Work out the finished part from the listing and answer in its coordinate system (mm). Face numbers are marked on the shaded views. A direction names the side the tool comes from. Give positions to 0.01 mm unless a question says otherwise; leave off trailing zeros. Loops run counter-clockwise (first coordinate to the right, second up) from the corner with the lowest first, then second, coordinate; pieces in that order, holes last. Notation, with made-up numbers: (18, 79.5) - (72, 79.5) arc R21 cw to (72, 116.5) - close; hole circle Ø3 at (-6, 4.5). An arc over 180 degrees is marked (long way). One line per item, written item: value.
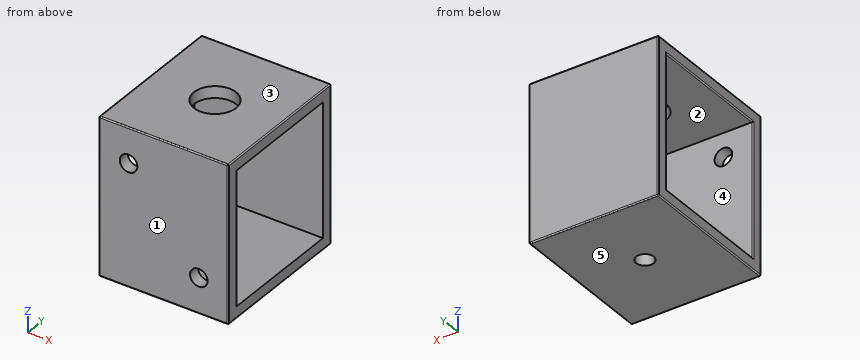
Autodesk Inventor part; units mm, degrees
ref_plane "YZ Plane" through (0, 0, 0) normal (1, 0, 0) x (0, 1, 0)
ref_plane "XZ Plane" through (0, 0, 0) normal (0, 1, 0) x (-1, 0, 0)
ref_plane "XY Plane" through (0, 0, 0) normal (0, 0, 1) x (1, 0, 0)
sketch "Sketch1" plane through (0, 0, 0) normal (0, 1, 0) x (-1, 0, 0)
  line L0 (11.5005, 11.58) -> (-10.5995, 11.58)
  line L1 (-10.5995, 11.58) -> (-10.5995, -15.22)
  line L2 (-10.5995, -15.22) -> (11.5005, -15.22)
  line L3 (11.5005, -15.22) -> (11.5005, 11.58)
  point P0 (0, 0)
  dimension "d0" = 22.1
  dimension "d1" = 26.8
extrude "Extrusion1" add sketch "Sketch1" along normal blind 25.4
shell "Shell1" thickness 2 removed faces 2 at (-11.5005, 8.4667, -6.2867) at (10.5995, 8.4667, 2.6466)
sketch "Sketch2" plane through (0, 0, 0) normal (0, -1, 0) x (1, 0, 0)
  line L0 (-11.5005, 11.58) -> (10.5995, 11.58)
  line L1 (-0.4505, 11.58) -> (-0.4505, -15.22)
  line L2 (10.5995, -15.22) -> (-11.5005, -15.22)
  circle A0 centre (-0.4505, -1.82) radius 9.5
  circle A1 centre (-6.4505, 5.5454) radius 1.5
  circle A2 centre (5.5495, -9.1855) radius 1.5
  point P0 (0, 0)
  dimension "d4" = 19
  dimension "d5" = 3
  dimension "d6" = 3
  dimension "d7" = 6
  dimension "d8" = 12
extrude "Extrusion2" cut sketch "Sketch2" against normal up to next contours A1 A0 | A0 A1 | A2 A0 | A0 A2
sketch "Sketch3" plane through (-11.5005, 0, 11.58) normal (0, 0, 1) x (1, 0, 0)
  line L0 (22.1, 0) -> (0, 0)
  line L1 (11.05, 0) -> (11.05, 25.4)
  line L2 (0, 25.4) -> (22.1, 25.4)
  circle A0 centre (11.05, 12.7) radius 3.6
  point P0 (11.5005, 0)
  dimension "d12" = 7.2
extrude "Extrusion3" cut sketch "Sketch3" against normal up to next
sketch "Sketch4" plane through (10.5995, 0, -15.22) normal (0, 0, -1) x (-1, 0, 0)
  line L0 (0, 25.4) -> (22.1, 25.4)
  line L1 (11.05, 25.4) -> (11.05, 0)
  line L2 (22.1, 0) -> (0, 0)
  circle A0 centre (11.05, 12.7) radius 1.5
  point P0 (10.5995, 0)
  dimension "d15" = 3
extrude "Extrusion4" cut sketch "Sketch4" against normal up to next
fillet "Fillet1" radius 0.2 16 edges at (-11.5005, 12.7, 11.58) (-0.4505, 0, 11.58) (10.5995, 12.7, 11.58) (10.5995, 0, -1.82) (-11.5005, 0, -1.82) (-0.4505, 0, -15.22) (10.5995, 12.7, -15.22) (-11.5005, 12.7, -15.22) (-0.4505, 25.4, -15.22) (-11.5005, 25.4, -1.82) (-0.4505, 25.4, 11.58) (10.5995, 25.4, -1.82) (-11.5005, 12.7, -13.22) (-11.5005, 2, -1.82) (-11.5005, 12.7, 9.58) (-11.5005, 23.4, -1.82)
properties part number "Solenoid_shell"
1. Section A-A (y = 12.7) is taken. Write down the section's boundary in (x, z).
Output:
outline: (-11.5, -15.02) arc R0.2 ccw to (-11.3, -15.22) - (-1.95, -15.22) - (-1.95, -13.22) - (-11.3, -13.22) arc R0.2 ccw to (-11.5, -13.42) - close; (-11.5, 9.78) arc R0.2 ccw to (-11.3, 9.58) - (-4.05, 9.58) - (-4.05, 11.58) - (-11.3, 11.58) arc R0.2 ccw to (-11.5, 11.38) - close; (1.05, -15.22) - (10.4, -15.22) arc R0.2 ccw to (10.6, -15.02) - (10.6, -13.22) - (1.05, -13.22) - close; (3.15, 9.58) - (10.6, 9.58) - (10.6, 11.38) arc R0.2 ccw to (10.4, 11.58) - (3.15, 11.58) - close
2. The mould has two halves that part along Z. Classify the marked faces 1, 2 and 3: released by +Z, released by -Z, zero draft, split by the parting line, or undercut.
Output:
face 1: zero draft
face 2: undercut
face 3: released by +Z
3. For the marked faces 4 and 5, determine the directions among +Z, -Z, +X, -X, +Y, -Y from which every point of the face is accessible in a straight line to the end or side of a thin tool.
Output:
face 4: +X, -X
face 5: -Z, +X, -X, +Y, -Y
4. Section C-C (x = 3.5) is taken. Write down the section's boundary in (y, z), and give its area (3 significant figures).
Output:
outline: (0, -15.02) arc R0.2 ccw to (0.2, -15.22) - (25.2, -15.22) arc R0.2 ccw to (25.4, -15.02) - (25.4, 11.38) arc R0.2 ccw to (25.2, 11.58) - (0.2, 11.58) arc R0.2 ccw to (0, 11.38) - close; hole (2, -13.22) - (23.4, -13.22) - (23.4, 9.58) - (2, 9.58) - close
area: 193 mm²
5. Section D-D (y = 18.25) is taken. Write down the section's boundary in (x, z), and give its area (3 significant figures).
Output:
outline: (-11.5, -15.02) arc R0.2 ccw to (-11.3, -15.22) - (10.4, -15.22) arc R0.2 ccw to (10.6, -15.02) - (10.6, -13.22) - (-11.3, -13.22) arc R0.2 ccw to (-11.5, -13.42) - close; (-11.5, 9.78) arc R0.2 ccw to (-11.3, 9.58) - (10.6, 9.58) - (10.6, 11.38) arc R0.2 ccw to (10.4, 11.58) - (-11.3, 11.58) arc R0.2 ccw to (-11.5, 11.38) - close
area: 88.3 mm²
6. Section B-B (z = -12) is taken. Write down the section's boundary in (x, y), and give its area (3 significant figures).
Output:
outline: (-11.5, 0.2) arc R0.2 ccw to (-11.3, 0) - (10.4, 0) arc R0.2 ccw to (10.6, 0.2) - (10.6, 2) - (-11.3, 2) arc R0.2 ccw to (-11.5, 1.8) - close; (-11.5, 23.6) arc R0.2 ccw to (-11.3, 23.4) - (10.6, 23.4) - (10.6, 25.2) arc R0.2 ccw to (10.4, 25.4) - (-11.3, 25.4) arc R0.2 ccw to (-11.5, 25.2) - close
area: 88.3 mm²
7. Flat-ended cylindrical pins translate along their axes: pin 1 Ø6.5 at (x, y) = (-0.45, 12.7) entering from -Z; pin 2 Ø2.5 at (x, y) = (-0.45, 12.7) entering from +Z; pin 3 Ø2.5 at (x, z) = (5.55, -9.19) entering from -Y. Find the tip coordinate at first contact, or state that the pin passes through.
Output:
pin 1: stops at z = -15.22
pin 2: passes through
pin 3: stops at y = 23.4
8. Find the intervals of material crossed by line 1 along Z through (x, y) = (-5.75, 19.5); line 2 along Y through (x, z) = (-3, -6.75); line 3 along X through (y, z) = (12.7, -14.6), in increasing order.
Output:
line 1: z = -15.22 to -13.22, 9.58 to 11.58
line 2: y = 0 to 2, 23.4 to 25.4
line 3: x = -11.5 to -1.95, 1.05 to 10.6
